Read the model definition and answer for the solid it produces. Units are mm, in the model's axes. Face numbers are marked on the shaded views. A direction names the side the tool comes from. Coordinates: 2 decimals unless noted, no trailing zeros. Order: outer loops, then holes, each group sorted by start corner. A loop starts at its lowest first (then second) coordinate and runs counter-clockwise, first axis right, second up. Notation, with made-up numbers: (79.25, 49) - (89.25, 49) arc R9 ccw to (89.25, 53) - close; hole circle Ø1 at (82.5, 3.25). An arc over 180 degrees is marked (long way). Write item = value, one per line.
Autodesk Inventor part; units mm, degrees
ref_plane "YZ Plane" through (0, 0, 0) normal (1, 0, 0) x (0, 1, 0)
ref_plane "XZ Plane" through (0, 0, 0) normal (0, 1, 0) x (-1, 0, 0)
ref_plane "XY Plane" through (0, 0, 0) normal (0, 0, 1) x (1, 0, 0)
sketch "Sketch1" plane through (0, 0, 0) normal (0, 1, 0) x (-1, 0, 0)
  line L0 (0, 0) -> (-21, 0)
  line L1 (-21, 0) -> (-21, 46)
  line L2 (-21, 46) -> (0, 46)
  line L3 (0, 46) -> (0, 0)
  dimension "d0" = 21
  dimension "d1" = 46
extrude "Extrusion1" add sketch "Sketch1" along normal blind 3
sketch "Sketch2" plane through (0, 3, 0) normal (0, 1, 0) x (1, 0, 0)
  line L0 (21, 0) -> (0, 0)
  line L1 (0, -46) -> (21, -46)
  circle A0 centre (10.5, -39.5) radius 6
  line L2 (0, 0) -> (0, -46)
  line L3 (0, -23) -> (21, -23)
  line L4 (21, -46) -> (21, 0)
  circle A1 centre (10.5, -6.5) radius 6
  dimension "d6" = 12
extrude "Extrusion2" add sketch "Sketch2" along normal blind 12 contours A0 | A1
sketch "Sketch3" plane through (0, 0, 0) normal (-1, 0, 0) x (0, 0, 1)
  line L0 (46, 0) -> (0, 0)
  line L1 (18, 0) -> (28, 0)
  line L2 (28, 0) -> (28, -4.5)
  line L3 (28, -4.5) -> (18, -4.5)
  line L4 (18, -4.5) -> (18, 0)
  dimension "d11" = 10
extrude "Extrusion3" add sketch "Sketch3" along normal blind 6
sketch "Sketch4" plane through (0, 0, 0) normal (1, 0, 0) x (0, 0, -1)
  line L0 (-28, -4.5) -> (-28, 0)
  line L1 (-18, 0) -> (-18, -4.5)
  line L2 (-28, 0) -> (-18, 0)
  line L3 (-18, 0) -> (-18, -4.5)
  line L4 (-18, -4.5) -> (-28, -4.5)
  line L5 (-28, -4.5) -> (-28, 0)
  point P0 (0, 0)
extrude "Extrusion4" add sketch "Sketch4" along normal blind 2
properties part number "Sensore ultrasuoni"
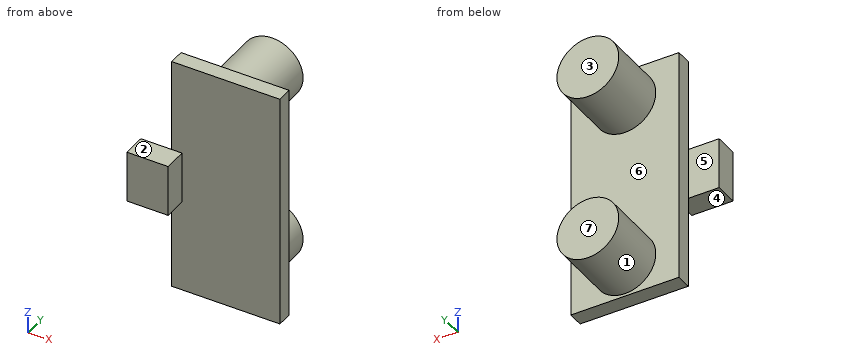
1) Determine the mould class of the marked faces 1, 2, 3 and 4 for opening direction Z: pulls with the +Z half, pulls with the -Z half, needs draft (parallel to the pull), parting line crosses it, or undercut.
Returned:
face_1 = undercut
face_2 = pulls with the +Z half
face_3 = needs draft
face_4 = pulls with the -Z half
2) For the marked faces 5, 6 and 7, determine the directions among +Z, -Z, +X, -X, +Y, -Y from which every point of the face is accessible in a straight line to the end or side of a thin tool.
Returned:
face_5 = +Z, -Z, -X, +Y
face_6 = +Y
face_7 = +Z, -Z, +X, -X, +Y
3) The part is cut by section A-A (z = 39.5). Determine the outline of the cut face in (x, y).
Returned:
outline = (0, 0) - (21, 0) - (21, 3) - (16.5, 3) - (16.5, 15) - (4.5, 15) - (4.5, 3) - (0, 3) - close
4) The part is cut by section C-C (x = 10.5). Determine the outline of the cut face in (y, z), and give its area (3 significant figures).
Returned:
outline = (0, 0) - (3, 0) - (3, 0.5) - (15, 0.5) - (15, 12.5) - (3, 12.5) - (3, 33.5) - (15, 33.5) - (15, 45.5) - (3, 45.5) - (3, 46) - (0, 46) - close
area = 426 mm^2
5) Flat-ended cylindrical pins translate along their axes: pin 1 Ø6 at (x, y) = (17, 5) entering from -Z; pin 2 Ø4 at (x, z) = (9.5, 21.5) entering from -Y; pin 3 Ø3.5 at (y, z) = (1, 15) entering from -X; pin 4 Ø1 at (x, y) = (12.5, 11) entering from +Z. Find the tip coordinate at first contact, or state that the pin passes through.
Returned:
pin_1 = 0
pin_2 = 0
pin_3 = 0
pin_4 = 45.31
6) Straight lines are drawn through the part: line 1 along Z through (x, y) = (10.5, 5); line 2 along Y through (x, z) = (15, 8.5); line 3 along Y through (x, z) = (9.25, 28.5). For each, find the intervals that lie inside material, in ascending order. Write a range as from..to.
Returned:
line_1 = 0.5..12.5, 33.5..45.5
line_2 = 0..15
line_3 = 0..3
7) The part is cut by section D-D (z = 19). Determine the outline of the cut face in (x, y).
Returned:
outline = (-6, -4.5) - (2, -4.5) - (2, 0) - (21, 0) - (21, 3) - (0, 3) - (0, 0) - (-6, 0) - close
8) The part is cut by section B-B (y = 8.5). Determine the outline of the cut face in (x, z).
Returned:
outline = circle Ø12 at (10.5, 6.5); circle Ø12 at (10.5, 39.5)
